Here's how the part is built. I have some questions about the finished solid (model axes, mm). A direction names the side the tool comes from. Give positions to 0.01 mm unless a question says otherwise; leave off trailing zeros. Loops run counter-clockwise (first coordinate to the right, second up) from the corner with the lowest first, then second, coordinate; pieces in that order, holes last. Notation, with made-up numbers: (22, -8) -> (41, -8) arc R20 cw to (41, 12) -> close; hole circle Ø11 at (50, 0). An arc over 180 degrees is marked (long way). Answer in a Markdown table with one row per item. Add a question column.
Item 1: If I drill on line 1 (Y direction, x = 5, z = 1.6); line 2 (Y direction, x = 12.5, z = 0.9); line 3 (X direction, y = 4.25, z = 0.35), over which ranges is the centre line in solid material (lowest first)?
Item 2: We'd pull the mould along X, two halves only. Please class faces 6 (the face through (3.5, 10, 1)), 7 (the face through (13, 15, 1)), 8 (the face through (-5, 21, 1)): released by +X, released by -X, zero draft, split by the parting line, or undercut.
Item 3: Which directions (+Z, -Z, +X, -X, +Y, -Y) give clear straight access to the entire face, cutting with the end or side of a thin tool? Please do faces 1 (the face through (6.5, 11, 1)), 2 (the face through (0, 6, 1)), 3 (the face through (10, 6, 1)), 4 (the face through (7, 15, 2)), 5 (the face through (5, 0, 1)).
Item 4: If we section it at B-B (y = 23.5): Write out the boundary of the cut face in (x, z), then the cut area to 3 significant figures.
Item 5: If we section it at C-C (z = 1.15): Write out the boundary of the cut face in (x, y).
Item 6: If we section it at A-A (x = -3): Write out the boundary of the cut face in (y, z).
Item 7: For P1, Ø1, axis at y = 10.5, z = 0.5, coming from the -X side; P2, Ø0.6, axis at y = 12, z = 1.5, coming from the +X side; P3, Ø1.5, axis at x = -3, y = 23.5, coming from the +Z side; P4, Ø1, axis at y = 7.5, z = 1, coming from the +X side, each with a flat end and sliding along its axis, tell me the tip position at first contact or that it passes through.
```python
from build123d import *

# Parameters (mm, degrees)
SKETCH1_W           = 10
SKETCH1_H           = 30
BOSS_EXTRUDE1_DEPTH = 2
SKETCH2_R           = 2.5
CUT_EXTRUDE1_DEPTH  = 2
CUT_EXTRUDE2_DEPTH  = 2
BOSS_EXTRUDE2_DEPTH = 2
SKETCH5_R           = 1.25
CUT_EXTRUDE3_DEPTH  = 2


with BuildPart() as part:
    # Sketch1 → Boss-Extrude1 (new body)
    with BuildSketch(Plane.XY):
        with Locations((5, 15)):
            Rectangle(SKETCH1_W, SKETCH1_H)
    extrude(amount=BOSS_EXTRUDE1_DEPTH)

    # Sketch2 → Cut-Extrude1 (cut)
    with BuildSketch(Plane.XY.offset(2)):
        with Locations((5, 25)):
            Circle(SKETCH2_R)
    extrude(amount=-CUT_EXTRUDE1_DEPTH, mode=Mode.SUBTRACT)

    # Sketch3 → Cut-Extrude2 (cut)
    with BuildSketch(Plane.XY.offset(2)):
        with BuildLine():
            Line((3.5, 3), (3.5, 18))
            ThreePointArc((3.5, 18), (5, 19.5), (6.5, 18))
            Line((6.5, 18), (6.5, 3))
            ThreePointArc((6.5, 3), (5, 1.5), (3.5, 3))
        make_face()
    extrude(amount=-CUT_EXTRUDE2_DEPTH, mode=Mode.SUBTRACT)

    # Sketch4 → Boss-Extrude2 (add)
    with BuildSketch(Plane.XY.offset(2)):
        Polygon((0, 30), (-5, 25), (-5, 17), (0, 12), align=None)
        Polygon((10, 30), (15, 25), (15, 17), (10, 12), align=None)
    extrude(amount=-BOSS_EXTRUDE2_DEPTH)

    # Sketch5 → Cut-Extrude3 (cut)
    with BuildSketch(Plane.XY.offset(2)):
        with Locations((-3, 23.5)):
            Circle(SKETCH5_R)
        with Locations((-3, 18.5)):
            Circle(SKETCH5_R)
        with Locations((13, 18.5)):
            Circle(SKETCH5_R)
        with Locations((13, 23.5)):
            Circle(SKETCH5_R)
    extrude(amount=-CUT_EXTRUDE3_DEPTH, mode=Mode.SUBTRACT)


solid = part.part
```
Recorded:
| question | item | result |
|---|---|---|
| 1 | line 1 | y = 0 to 1.5, 19.5 to 22.5, 27.5 to 30 |
| 1 | line 2 | y = 14.5 to 17.35, 19.65 to 22.35, 24.65 to 27.5 |
| 1 | line 3 | x = 0 to 3.5, 6.5 to 10 |
| 2 | face 6 | undercut |
| 2 | face 7 | released by +X |
| 2 | face 8 | released by -X |
| 3 | face 1 | +Z, -Z |
| 3 | face 2 | +Z, -Z, -X, -Y |
| 3 | face 3 | +Z, -Z, +X, -Y |
| 3 | face 4 | +Z, +X, -X, +Y, -Y |
| 3 | face 5 | +Z, -Z, +X, -X, -Y |
| 4 | outline | (-5, 0) -> (-4.25, 0) -> (-4.25, 2) -> (-5, 2) -> close; (-1.75, 0) -> (3, 0) -> (3, 2) -> (-1.75, 2) -> close; (7, 0) -> (11.75, 0) -> (11.75, 2) -> (7, 2) -> close; (14.25, 0) -> (15, 0) -> (15, 2) -> (14.25, 2) -> close |
| 4 | area | 22.0 mm^2 |
| 5 | outline | (-5, 17) -> (0, 12) -> (0, 0) -> (10, 0) -> (10, 12) -> (15, 17) -> (15, 25) -> (10, 30) -> (0, 30) -> (-5, 25) -> close; hole circle Ø2.5 at (-3, 18.5); hole circle Ø2.5 at (-3, 23.5); hole circle Ø5 at (5, 25); hole (3.5, 3) arc R1.5 ccw to (6.5, 3) -> (6.5, 18) arc R1.5 ccw to (3.5, 18) -> close; hole circle Ø2.5 at (13, 18.5); hole circle Ø2.5 at (13, 23.5) |
| 6 | outline | (15, 0) -> (17.25, 0) -> (17.25, 2) -> (15, 2) -> close; (19.75, 0) -> (22.25, 0) -> (22.25, 2) -> (19.75, 2) -> close; (24.75, 0) -> (27, 0) -> (27, 2) -> (24.75, 2) -> close |
| 7 | P1 | stops at x = 0 |
| 7 | P2 | stops at x = 10.3 |
| 7 | P3 | passes through |
| 7 | P4 | stops at x = 10 |
